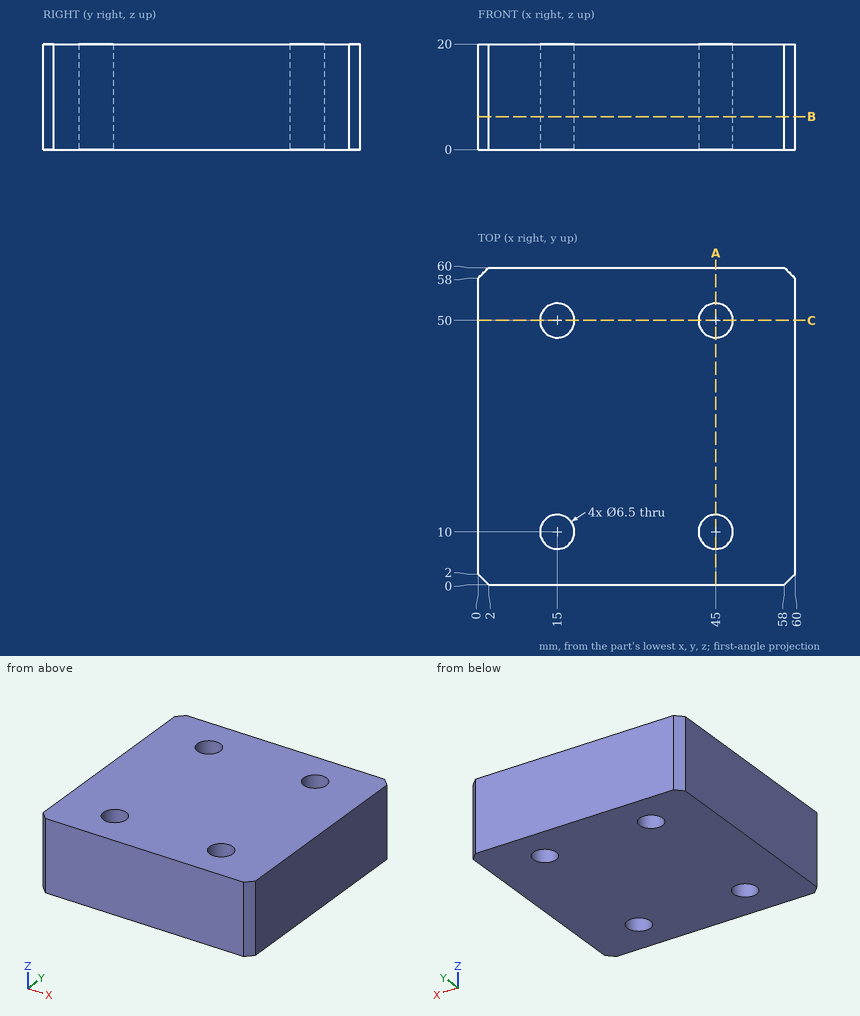
Can you work these out from the drawing? Everything is in mm from the part's minimum corner. Round coordinates to 2 decimals unless told otherwise and drop trailing zeros. Order: outer loops, then holes, each group sorted by start corner. A loop starts at its lowest first (then second) coordinate and runs counter-clockwise, first axis right, second up. Notation, with made-up numbers: (54, -6.5) -> (87, -6.5) arc R5 cw to (87, -2.5) -> close; hole circle Ø8 at (44, -12.75). An arc over 180 degrees is marked (long way). Return JSON: item names as keys, results as strings. Group by question number.
1. If we section it at C-C, the plane y = 50: Write out the boundary of the cut face in (x, z), then the cut area to 3 significant figures.
2. If we section it at B-B, the plane z = 6.25: Write out the boundary of the cut face in (x, y).
3. If we section it at A-A, the plane x = 45: Write out the boundary of the cut face in (y, z).
4. Will this pin go through, and if not, where does the flat tip stop? pin 1 (6 mm diameter, centred on x = 15, y = 10, fed in from +Z).
5. I need wall thicknesses on line 1 (Y direction, x = 45, z = 5.5); line 2 (Y direction, x = 13, z = 6.25); line 3 (X direction, y = 53, z = 15.5). Which ranges of each line are inside material? Lowest first, please. Write a range as [from, to].
Output values:
{
 "1": {"outline": "(0, 0) -> (11.75, 0) -> (11.75, 20) -> (0, 20) -> close; (18.25, 0) -> (41.75, 0) -> (41.75, 20) -> (18.25, 20) -> close; (48.25, 0) -> (60, 0) -> (60, 20) -> (48.25, 20) -> close", "area": "940 mm²"},
 "2": {"outline": "(0, 2) -> (2, 0) -> (58, 0) -> (60, 2) -> (60, 58) -> (58, 60) -> (2, 60) -> (0, 58) -> close; hole circle Ø6.5 at (15, 10); hole circle Ø6.5 at (15, 50); hole circle Ø6.5 at (45, 10); hole circle Ø6.5 at (45, 50)"},
 "3": {"outline": "(0, 0) -> (6.75, 0) -> (6.75, 20) -> (0, 20) -> close; (13.25, 0) -> (46.75, 0) -> (46.75, 20) -> (13.25, 20) -> close; (53.25, 0) -> (60, 0) -> (60, 20) -> (53.25, 20) -> close"},
 "4": {"pin 1": "through"},
 "5": {"line 1": "[0, 6.75], [13.25, 46.75], [53.25, 60]", "line 2": "[0, 7.44], [12.56, 47.44], [52.56, 60]", "line 3": "[0, 13.75], [16.25, 43.75], [46.25, 60]"}
}
